The model under review builds one solid part; all positions refer to its coordinate system, in mm. A direction names the side the tool comes from. Coordinates: 2 decimals unless noted, no trailing zeros. Write each loop counter-clockwise with the first axis right and the second up, starting at its lowest first coordinate (ties: lowest second). Pieces come first, ordered by that corner, then holes.
1) Machinability: for faces 1 (the flat face through (-60, -3, 2.77)), 2 (the cylindrical face through (79.664, -11.761, -11.128)), 3 (the flat face through (-67.31, -3, 7)), which of the approach directions +Z, -Z, +X, -X, +Y, -Y give a long, thin tool a straight path to every point of the face, cutting with its end or side? Answer none if there is none.
2) Mouldability with a two-part tool opening along Z and no side actions: class faces 4 (the flat face through (72.39, -3, 7)), 5 (the cylindrical face through (-81.088, -11.761, 28.686)), 6 (the flat face through (65, -3, 2.77)) as released by +Z, released by -Z, zero draft, split by the parting line, or undercut.
3) Add section A-A, the plane z = -2.5. State the section outline as (x, y) points.
4) For P1, Ø2.5, axis at x = 75.5, z = 26, coming from the -Y side (3 decimals); P2, Ø0.8, axis at x = 71, y = -3, coming from the +Z side; P3, Ø12, axis at x = -77.72, z = 25.6, coming from the +Y side, all flat-tipped, find the tip position at first contact; note any pin that passes through.
5) For line 1 (X direction, y = -2.75, z = 14); line 2 (Z direction, x = 79.5, y = -11.5); line 3 (Z direction, x = -64, y = -2), list the stretches that pass through material, from the lowest coordinate up.
6) Add section B-B, the plane y = -4. State the section outline as (x, z) points.
7) Add section C-C, the plane x = 76. State the section outline as (y, z) points (3 decimals), then the cut area to 3 significant figures.
8) Add section D-D, the plane z = 9.5. State the section outline as (x, y) points.
from build123d import *

# Parameters (mm, degrees)
F1_DEPTH = 12.7
F2_R     = 4.564063
F3_DEPTH = 1.905
F4_W     = 31.75
F4_H     = 63.5
F5_DEPTH = 6.35
F6_W     = 2.7686
F6_H     = 6.35
F7_DEPTH = 2.9972
F8_DEPTH = 38.1


with BuildPart() as f1:
    # F0 (on Front) → F1 (new body)
    with BuildSketch(Plane.XZ):
        Polygon((104.14, 40.870185), (2.54, 40.870185), (-99.06, 40.870185), (-99.06, -22.629815), (2.54, -22.629815), (104.14, -22.629815), align=None)
    extrude(amount=F1_DEPTH)

    # F2 (on face) → F3 (cut)
    with BuildSketch(Plane.XZ.offset(12.7)):
        with Locations((-77.724032, -12.498807)):
            Circle(F2_R)
        with Locations((75.310968, -12.498807)):
            Circle(F2_R)
        with Locations((75.310968, 25.601193)):
            Circle(F2_R)
        with Locations((-77.724032, 25.601193)):
            Circle(F2_R)
    extrude(amount=-F3_DEPTH, mode=Mode.SUBTRACT)

    # F4 (on face) → F5 (cut)
    with BuildSketch(Plane(origin=(0, 0, 0), x_dir=(-1, 0, 0), z_dir=(0, 1, 0))):
        with Locations((-88.265, 9.120185)):
            Rectangle(F4_W, F4_H)
        with Locations((83.185, 9.120185)):
            Rectangle(F4_W, F4_H)
    extrude(amount=-F5_DEPTH, mode=Mode.SUBTRACT)

    # F6 (on face) → F7 (cut)
    with BuildSketch(Plane.XY.offset(40.870185)):
        with Locations((-65.9257, -3.175)):
            Rectangle(F6_W, F6_H)
        Polygon((-64.5414, 0), (-64.5414, -6.35), (-57.3786, -6.35), (-54.61, -6.35), (-54.61, 0), (-57.3786, 0), align=None)
        with Locations((71.0057, -3.175)):
            Rectangle(F6_W, F6_H)
        Polygon((62.4586, -6.35), (69.6214, -6.35), (69.6214, 0), (62.4586, 0), (59.69, 0), (59.69, -6.35), align=None)
    extrude(amount=-F7_DEPTH, mode=Mode.SUBTRACT)

    # F6 (on face) → F8 (cut)
    with BuildSketch(Plane.XY.offset(40.870185)):
        Polygon((-64.5414, 0), (-64.5414, -6.35), (-57.3786, -6.35), (-54.61, -6.35), (-54.61, 0), (-57.3786, 0), align=None)
        Polygon((62.4586, 0), (59.69, 0), (59.69, -6.35), (62.4586, -6.35), (69.6214, -6.35), (69.6214, 0), align=None)
    extrude(amount=-F8_DEPTH, mode=Mode.SUBTRACT)


solid = f1.part
Geometry results:
1. face 1: +Z, +Y
1. face 2: -Y
1. face 3: +Z, -Z, -X, +Y
2. face 4: zero draft
2. face 5: undercut
2. face 6: released by +Z
3. outline: (-99.06, -12.7) - (104.14, -12.7) - (104.14, -6.35) - (72.39, -6.35) - (72.39, 0) - (-67.31, 0) - (-67.31, -6.35) - (-99.06, -6.35) - close
4. P1: stops at y = -10.795
4. P2: stops at z = 37.87
4. P3: stops at y = -6.35
5. line 1: x = -67.31 to -64.54, -54.61 to 59.69, 69.62 to 72.39
5. line 2: z = -22.63 to -14.31, -10.69 to 23.79, 27.41 to 40.87
5. line 3: z = -22.63 to 2.77
6. outline: (-67.31, -22.63) - (72.39, -22.63) - (72.39, 37.87) - (69.62, 37.87) - (69.62, 2.77) - (59.69, 2.77) - (59.69, 40.87) - (-54.61, 40.87) - (-54.61, 2.77) - (-64.54, 2.77) - (-64.54, 37.87) - (-67.31, 37.87) - close
7. outline: (-12.7, -22.63) - (-6.35, -22.63) - (-6.35, 40.87) - (-12.7, 40.87) - (-12.7, 30.113) - (-10.795, 30.113) - (-10.795, 21.089) - (-12.7, 21.089) - (-12.7, -7.987) - (-10.795, -7.987) - (-10.795, -17.011) - (-12.7, -17.011) - close
7. area: 369 mm2
8. outline: (-99.06, -12.7) - (104.14, -12.7) - (104.14, -6.35) - (72.39, -6.35) - (72.39, 0) - (69.62, 0) - (69.62, -6.35) - (59.69, -6.35) - (59.69, 0) - (-54.61, 0) - (-54.61, -6.35) - (-64.54, -6.35) - (-64.54, 0) - (-67.31, 0) - (-67.31, -6.35) - (-99.06, -6.35) - close
